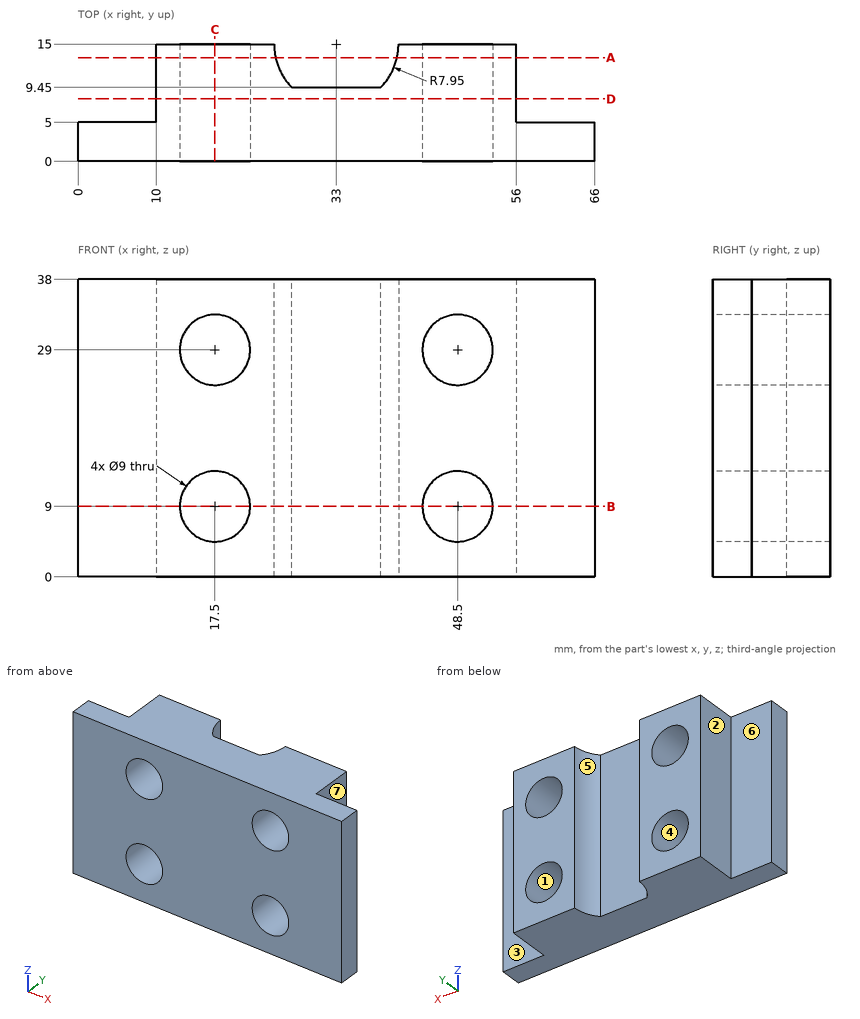
Answer from the drawing. Dimensions are ordinates in mm from the lowest x, y and z of the part. A direction names the side the tool comes from. Give positions to 0.01 mm unless a question says otherwise; leave off trailing zeros. Loops run counter-clockwise (first coordinate to the right, second up) from the corner with the lowest first, then second, coordinate; pieces in that order, holes last. Notation, with made-up numbers: (46.25, 71) -> (58.25, 71) arc R13 ccw to (58.25, 93) -> close; hole circle Ø7 at (79.25, -40). An arc over 180 degrees is marked (long way). One line per question, with ' | ' between items. Start each with the question number.
1) Each of these flat-tipped pins is pushed along its axis until it touches: pin 1 (11 mm diameter, centred on x = 62.5, z = 17, fed in from +Y); pin 2 (8 mm diameter, centred on x = 8.5, y = 4, fed in from -Z); pin 3 (3.5 mm diameter, centred on x = 30.5, z = 22, fed in from +Y); pin 4 (1 mm diameter, centred on y = 10.5, z = 18.5, fed in from -X). Where does it stop, or does it pass through?
2) Section D-D, the plane y = 8 is taken. Determine the outline of the cut face in (x, z), then the cut area to 3 significant figures.
3) Straight lines are drawn through the part: L1, parallel to X at y = 8, z = 9; L2, parallel to Z at x = 48.5, y = 5.25; L3, parallel to X at y = 12, z = 29. For each, find the intervals that lie inside material, in ascending order.
4) Determine the mould class of the marked faces 1, 2, 3 and 4 for opening direction X: +X half, -X half, draft (parallel to the pull), parting line (faces both ways), or undercut.
5) Section A-A, the plane y = 13.25 is taken. Determine the outline of the cut face in (x, z) (3 decimals).
6) Section B-B, the plane z = 9 is taken. Determine the outline of the cut face in (x, y), then the cut area to 3 significant figures.
7) Section C-C, the plane x = 17.5 is taken. Determine the outline of the cut face in (y, z).
8) For the marked faces 5, 6 and 7, determine the directions among +Z, -Z, +X, -X, +Y, -Y from which every point of the face is accessible in a straight line to the end or side of a thin tool.
Resolved:
1) pin 1: y = 5 | pin 2: z = 0 | pin 3: y = 9.45 | pin 4: x = 10
2) outline: (10, 0) -> (56, 0) -> (56, 38) -> (10, 38) -> close; hole circle Ø9 at (17.5, 9); hole circle Ø9 at (17.5, 29); hole circle Ø9 at (48.5, 9); hole circle Ø9 at (48.5, 29) | area: 1,490 mm2
3) L1: 10 to 13, 22 to 44, 53 to 56 | L2: 0 to 4.5, 13.5 to 24.5, 33.5 to 38 | L3: 10 to 13, 22 to 25.64, 40.36 to 44, 53 to 56
4) face 1: undercut | face 2: -X half | face 3: draft | face 4: undercut
5) outline: (10, 0) -> (25.245, 0) -> (25.245, 38) -> (10, 38) -> close; (40.755, 0) -> (56, 0) -> (56, 38) -> (40.755, 38) -> close; hole circle Ø9 at (17.5, 9); hole circle Ø9 at (17.5, 29); hole circle Ø9 at (48.5, 9); hole circle Ø9 at (48.5, 29)
6) outline: (0, 0) -> (13, 0) -> (13, 15) -> (10, 15) -> (10, 5) -> (0, 5) -> close; (22, 0) -> (44, 0) -> (44, 15) -> (40.95, 15) arc R7.95 cw to (38.69, 9.45) -> (27.31, 9.45) arc R7.95 cw to (25.05, 15) -> (22, 15) -> close; (53, 0) -> (66, 0) -> (66, 5) -> (56, 5) -> (56, 15) -> (53, 15) -> close | area: 440 mm2
7) outline: (0, 0) -> (15, 0) -> (15, 4.5) -> (0, 4.5) -> close; (0, 13.5) -> (15, 13.5) -> (15, 24.5) -> (0, 24.5) -> close; (0, 33.5) -> (15, 33.5) -> (15, 38) -> (0, 38) -> close
8) face 5: +Z, -Z, +Y | face 6: +Z, -Z, -X, +Y | face 7: +Z, -Z, +X, +Y
